```python
from build123d import *

# Parameters (mm, degrees)
F0_R     = 11
F1_DEPTH = 15
F2_DEPTH = 4
F3_R     = 5


with BuildPart() as f1:
    # F0 (on Front) → F1 (new body, symmetric)
    with BuildSketch(Plane.XZ):
        with BuildLine():
            Line((-55, 0), (0, 0))
            Line((0, 0), (55, 0))
            Line((55, 0), (55, 30))
            Line((55, 30), (47, 30))
            Line((47, 30), (47, 8))
            Line((47, 8), (20, 8))
            Line((20, 8), (20, 26))
            ThreePointArc((20, 26), (16.405315, 37.439651), (6.913438, 44.767109))
            ThreePointArc((6.913438, 44.767109), (3.511255, 45.689365), (0, 46))
            ThreePointArc((0, 46), (-3.511255, 45.689365), (-6.913438, 44.767109))
            ThreePointArc((-6.913438, 44.767109), (-16.405315, 37.439651), (-20, 26))
            Line((-20, 26), (-20, 8))
            Line((-20, 8), (-47, 8))
            Line((-47, 8), (-47, 30))
            Line((-47, 30), (-55, 30))
            Line((-55, 30), (-55, 0))
        make_face()
        with Locations((0, 26)):
            Circle(F0_R, mode=Mode.SUBTRACT)
    extrude(amount=F1_DEPTH, both=True)

    # F0 (on Front) → F2 (join, symmetric)
    with BuildSketch(Plane.XZ):
        with BuildLine():
            Line((-6.913438, 44.767109), (-47, 30))
            Line((-47, 30), (-47, 8))
            Line((-47, 8), (-20, 8))
            Line((-20, 8), (-20, 26))
            ThreePointArc((-20, 26), (-16.405315, 37.439651), (-6.913438, 44.767109))
        make_face()
        with BuildLine():
            Line((47, 8), (47, 30))
            Line((47, 30), (6.913438, 44.767109))
            ThreePointArc((6.913438, 44.767109), (16.405315, 37.439651), (20, 26))
            Line((20, 26), (20, 8))
            Line((20, 8), (47, 8))
        make_face()
    extrude(amount=F2_DEPTH, both=True)

    # F3
    f3_edges = [f1.edges().sort_by_distance(p)[0] for p in [
        (51, -15, 30),
        (-51, -15, 30),
        (-51, 15, 30),
        (51, 15, 30),
    ]]
    fillet(f3_edges, radius=F3_R)


solid = f1.part
```
Can you work these out from the model? Positions are in its coordinate system, mm. A direction names the side the tool comes from. Coordinates: 2 decimals unless noted, no trailing zeros. Order: outer loops, then holes, each group sorted by start corner. A loop starts at its lowest first (then second) coordinate and runs counter-clockwise, first axis right, second up. Notation, with made-up numbers: (76.5, -26.5) - (128.5, -26.5) arc R31 cw to (128.5, 8.5) - close; hole circle Ø2 at (-26, 32). An arc over 180 degrees is marked (long way). Answer in a Markdown table with one row per item.
1. For faces 4 (the cylindrical face through (-51, 14, 28)), 5 (the flat face through (-32, -4, 23)), 6 (the flat face through (-51, 0, 30)), 7 (the flat face through (51, 0, 30)), which set-ups out of +Z, -Z, +X, -X, +Y, -Y let a thin tool reach every point of the face, with its end or its side?
Reply:
| item | result |
|---|---|
| face 4 | +Z, -X, +Y |
| face 5 | +Z, -Y |
| face 6 | +Z, -X, +Y, -Y |
| face 7 | +Z, +X, +Y, -Y |
2. If we mould it in two halves opening along X, with no side actions, what happens to faces 1 (the flat face through (34, 9, 8)), 2 (the flat face through (55, 0, 15)), 3 (the cylindrical face through (51, 14, 28))? For each: pulls with the +X half, pulls with the -X half, needs draft (parallel to the pull), parting line crosses it, or undercut.
Reply:
| item | result |
|---|---|
| face 1 | undercut |
| face 2 | pulls with the +X half |
| face 3 | needs draft |
3. If I drill on line 1 along Z through (x, y) = (0, 0); line 2 along X through (y, z) = (-4.5, 27); line 3 along X through (y, z) = (8.25, 18), over which ranges is the centre line in solid material (lowest first)?
Reply:
| item | result |
|---|---|
| line 1 | z = 0 to 15, 37 to 46 |
| line 2 | x = -55 to -47, -19.97 to -10.95, 10.95 to 19.97, 47 to 55 |
| line 3 | x = -55 to -47, -20 to -7.55, 7.55 to 20, 47 to 55 |
4. Suppose I cut it at B-B (y = -0.25). Please give me the cut outline in (x, z).
Reply:
| item | result |
|---|---|
| outline | (-55, 0) - (55, 0) - (55, 30) - (47, 30) - (6.91, 44.77) arc R20 ccw to (0, 46) arc R20 ccw to (-6.91, 44.77) - (-47, 30) - (-55, 30) - close; hole circle Ø22 at (0, 26) |
5. Suppose I cut it at D-D (y = -5.5). Please give me the cut outline in (x, z).
Reply:
| item | result |
|---|---|
| outline | (-55, 0) - (55, 0) - (55, 30) - (47, 30) - (47, 8) - (20, 8) - (20, 26) arc R20 ccw to (6.91, 44.77) arc R20 ccw to (0, 46) arc R20 ccw to (-6.91, 44.77) arc R20 ccw to (-20, 26) - (-20, 8) - (-47, 8) - (-47, 30) - (-55, 30) - close; hole circle Ø22 at (0, 26) |
6. Suppose I cut it at A-A (z = 10.5). Please give me the cut outline in (x, y).
Reply:
| item | result |
|---|---|
| outline | (-55, -15) - (-47, -15) - (-47, -4) - (-20, -4) - (-20, -15) - (20, -15) - (20, -4) - (47, -4) - (47, -15) - (55, -15) - (55, 15) - (47, 15) - (47, 4) - (20, 4) - (20, 15) - (-20, 15) - (-20, 4) - (-47, 4) - (-47, 15) - (-55, 15) - close |
7. For pin 1 (3.5 mm diameter, centred on x = 36, y = -11, fed in from +Z); pin 2 (12 mm diameter, centred on x = -28, y = 7, fed in from +Z); pin 3 (9 mm diameter, centred on x = -49.5, y = -2.5, fed in from +Z); pin 4 (2 mm diameter, centred on x = -37.5, y = -2.5, fed in from -Z), each with a flat end and sliding along its axis, tell me the tip position at first contact or that it passes through.
Reply:
| item | result |
|---|---|
| pin 1 | stops at z = 8 |
| pin 2 | stops at z = 38.91 |
| pin 3 | stops at z = 30.74 |
| pin 4 | stops at z = 0 |
8. Suppose I cut it at C-C (x = 26.5). Please give me the cut outline in (y, z), and give its area (3 significant figures).
Reply:
| item | result |
|---|---|
| outline | (-15, 0) - (15, 0) - (15, 8) - (4, 8) - (4, 37.55) - (-4, 37.55) - (-4, 8) - (-15, 8) - close |
| area | 476 mm^2 |
